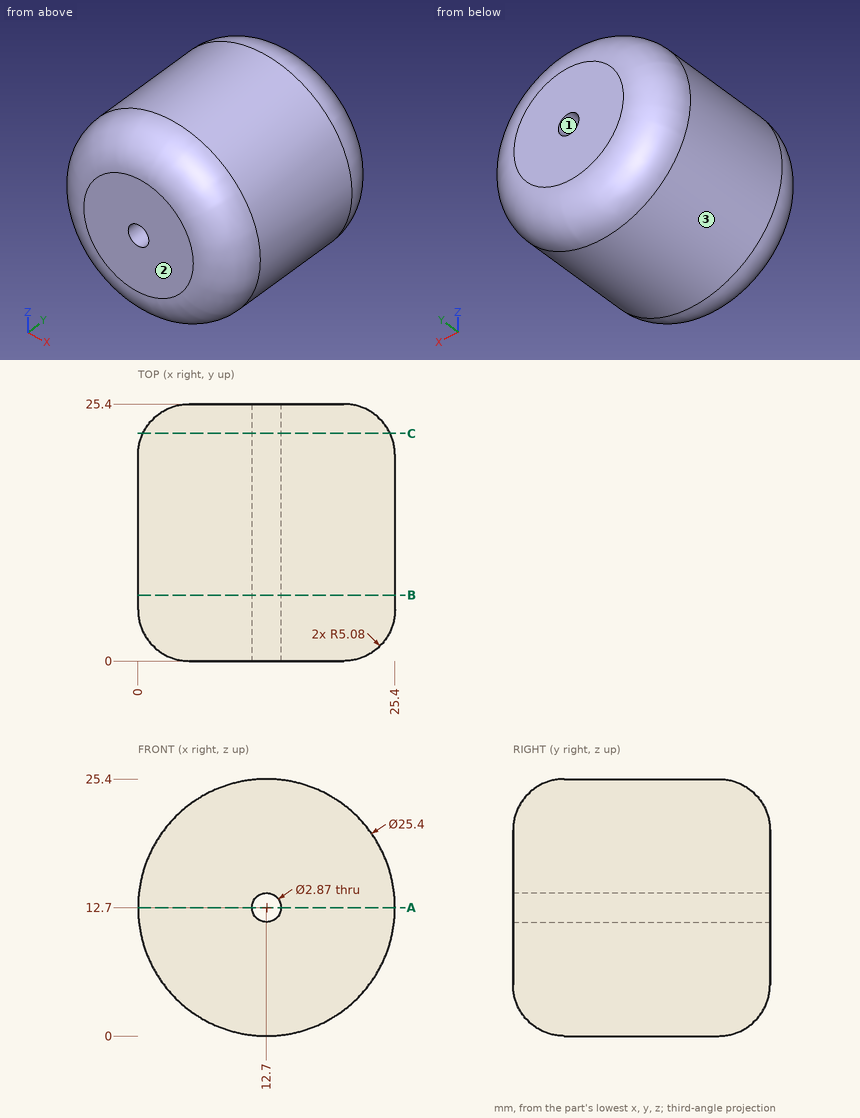
Here's the drawing with two shaded views (mm, measured from the low corner). I have some questions. Give positions to 0.01 mm unless a question says otherwise; leave off trailing zeros. Loops run counter-clockwise (first coordinate to the right, second up) from the corner with the lowest first, then second, coordinate; pieces in that order, holes last. Notation, with made-up numbers: M -11.75,26 L -5.75,26 A21 cw -5.75,56 Z; hole C 48.5,54.25 d9. An arc over 180 degrees is marked long. Use one line per item in the form item = value. Start each with the question number.
(1) I want a section at B-B, the plane y = 6.5. Write out the boundary of the cut face in (x, z) (1 decimal).
(2) Please list where these lines run through material, in increasing order: line 1 (Z direction, x = 12.7, y = 20) (1 decimal); line 2 (X direction, y = 20.25, z = 13.75); line 3 (Z direction, x = 14, y = 3.25).
(3) Thinking about a two-plate mould opening in X: for the marked faces 1, 2 and 3, which applies, released by +X, released by -X, zero draft, split by the parting line, or undercut?
(4) I'm going to push flat-ended pins straight in: P1, Ø2.5, axis at x = 12.7, z = 12.7, coming from the -Y side; P2, Ø12, axis at x = 5.5, y = 5, coming from the +Z side; P3, Ø8, axis at y = 8, z = 3, coming from the -X side; P4, Ø5, axis at y = 6.5, z = 10, coming from the -X side. Where does each tip first touch, or does it pass through?
(5) I want a section at A-A, the plane z = 12.7. Write out the boundary of the cut face in (x, y) (1 decimal).
(6) I want a section at C-C, the plane y = 22.5. Write out the boundary of the cut face in (x, z) (1 decimal).
Worked out:
q1.outline = C 12.7,12.7 d25.4; hole C 12.7,12.7 d2.9
q2.line_1 = 0 to 11.3, 14.1 to 25.4
q2.line_2 = 0.04 to 11.72, 13.68 to 25.36
q2.line_3 = 0.41 to 12.09, 13.31 to 24.99
q3.face_1 = undercut
q3.face_2 = zero draft
q3.face_3 = split by the parting line
q4.P1 = through
q4.P2 = 25.34
q4.P3 = 1.35
q4.P4 = 0
q5.outline = M 0,5.1 A5.1 ccw 5.1,0 L 11.3,0 L 11.3,25.4 L 5.1,25.4 A5.1 ccw 0,20.3 Z; M 14.1,0 L 20.3,0 A5.1 ccw 25.4,5.1 L 25.4,20.3 A5.1 ccw 20.3,25.4 L 14.1,25.4 Z
q6.outline = C 12.7,12.7 d24.4; hole C 12.7,12.7 d2.9
